Can you work these out from the model? Positions are in its coordinate system, mm. A direction names the side the tool comes from. Give positions to 0.01 mm unless a question says otherwise; leave off trailing zeros. Loops run counter-clockwise (first coordinate to the right, second up) from the corner with the lowest first, then second, coordinate; pieces in that order, holes last. Notation, with made-up numbers: (30.25, -28) -> (48.25, -28) arc R14 ccw to (48.25, -20) -> close; hole circle Ø5 at (-13.5, -8). An arc over 180 degrees is marked (long way). Use CSV: the item, a comma, the result in double quotes.
from build123d import *

# Parameters (mm, degrees)
SKETCH1_R           = 10.922
EXTRUDE1_DEPTH      = 94.869
EXTRUDE1_DEPTH_BACK = 94.869
SKETCH3_W           = 0.762
SKETCH3_H           = 0.762
RODHOLE_START       = -173.569
SKETCH8_R           = 3.175
RODHOLE_DEPTH       = 173.569
SKETCH9_R           = 9.525
STROKECHAMBER_DEPTH = 132
CHAMFER1_SIZE       = 0.5
SKETCH4_W           = 1.397
SKETCH4_H           = 12.7
SKETCH4_W_2         = 3.048
SKETCH4_H_2         = 3.048
FLATS_DEPTH         = 11.9220001
FLATS_DEPTH_BACK    = 11.9220001


with BuildPart() as part:
    # Sketch1 → Extrude1 (new body, two sides)
    with BuildSketch(Plane.XY) as extrude1_sk:
        Circle(SKETCH1_R)
    extrude(amount=EXTRUDE1_DEPTH)
    extrude(extrude1_sk.sketch, amount=-EXTRUDE1_DEPTH_BACK)

    # Sketch2 → Nose (revolve)
    with BuildSketch(Plane(origin=(0, 0, 0), x_dir=(0, 0, -1), z_dir=(1, 0, 0))):
        Polygon((-94.869, 7.9248), (-97.155, 7.9248), (-97.155, 7), (-99.955, 7), (-99.955, 7.9375), (-107.569, 7.9375), (-107.569, 0), (-94.869, 0), align=None)
    revolve(axis=Axis((0, 0, 0), (0, 0, 1)))

    # Sketch3 → CoverGrooves (revolve, cut)
    with BuildSketch(Plane(origin=(0, 0, 0), x_dir=(0, 0, -1), z_dir=(1, 0, 0))):
        with Locations((-75.438, 10.541)):
            Rectangle(SKETCH3_W, SKETCH3_H)
        Polygon((-74.295, 10.922), (-74.295, 10.16), (-73.533, 10.16), (-72.771, 10.922), align=None)
        Polygon((88.646, 10.922), (88.646, 10.16), (87.884, 10.922), align=None)
        Polygon((87.122, 10.922), (87.122, 10.16), (86.36, 10.922), align=None)
    revolve(axis=Axis((0, 0, 0), (0, 0, 1)), mode=Mode.SUBTRACT)

    # Sketch7 → FrontPort (revolve, cut)
    with BuildSketch(Plane(origin=(0, 0, 0), x_dir=(0, 0, -1), z_dir=(1, 0, 0))):
        Polygon((-83.439, 10.922), (-77.589, 10.922), (-78.289, 10.222), (-78.289, 0), (-83.439, 0), align=None)
    revolve(axis=Axis((0, 0, 83.439), (0, 1, 0)), mode=Mode.SUBTRACT)

    # Sketch8 → RodHole (cut)
    with BuildSketch(Plane.XY.offset(107.569).offset(RODHOLE_START)):
        Circle(SKETCH8_R)
    extrude(amount=RODHOLE_DEPTH, mode=Mode.SUBTRACT)

    # Sketch9 → StrokeChamber (cut)
    with BuildSketch(Plane.XY.offset(-66)):
        Circle(SKETCH9_R)
    extrude(amount=STROKECHAMBER_DEPTH, mode=Mode.SUBTRACT)

    # Chamfer1
    chamfer1_edges = [part.edges().sort_by_distance(p)[0] for p in [
        (-10.922, 0, -94.869),
        (-3.175, 0, 107.569),
        (0, -7.9375, 107.569),
        (-10.922, 0, 94.869),
    ]]
    chamfer(chamfer1_edges, length=CHAMFER1_SIZE)

    # Sketch4 → Flats (cut, two sides)
    with BuildSketch(Plane(origin=(0, 0, 0), x_dir=(1, 0, 0), z_dir=(0, 1, 0))) as flats_sk:
        with Locations((10.2235, -88.519)):
            Rectangle(SKETCH4_W, SKETCH4_H)
        with Locations((9.398, 93.345)):
            Rectangle(SKETCH4_W_2, SKETCH4_H_2)
        with Locations((-9.398, 93.345)):
            Rectangle(SKETCH4_W_2, SKETCH4_H_2)
        with Locations((-10.2235, -88.519)):
            Rectangle(SKETCH4_W, SKETCH4_H)
    extrude(amount=FLATS_DEPTH, mode=Mode.SUBTRACT)
    extrude(flats_sk.sketch, amount=-FLATS_DEPTH_BACK, mode=Mode.SUBTRACT)

    # Sketch10 → RearStdPort (revolve, cut)
    with BuildSketch(Plane(origin=(0, 0, 0), x_dir=(0, 0, -1), z_dir=(1, 0, 0))):
        Polygon((94.869, 0), (94.869, 5.85), (94.169, 5.15), (0, 5.15), (0, 0), align=None)
    revolve(axis=Axis((0, 0, 0), (0, 0, 1)), mode=Mode.SUBTRACT)


solid = part.part
(1) If we section it at C-C, the plane z = -33: Write out the boundary of the cut face in (x, y) (3 decimals), then the cut area to 3 significant figures.
Answer sheet:
outline,"circle Ø21.844 at (0, 0); hole circle Ø19.05 at (0, 0)"
area,"89.7 mm2"
(2) If we section it at D-D, the plane z = -73: Write out the boundary of the cut face in (x, y), then the cut area to 3 significant figures.
Answer sheet:
outline,"circle Ø21.84 at (0, 0); hole circle Ø10.3 at (0, 0)"
area,"291 mm2"
(3) If we section it at A-A, the plane z = 92: Write out the boundary of the cut face in (x, y) (3 decimals), then the cut area to 3 significant figures.
Answer sheet:
outline,"(-9.525, -5.345) arc R10.922 ccw to (9.525, -5.345) -> (9.525, 5.345) arc R10.922 ccw to (-9.525, 5.345) -> close; hole circle Ø6.35 at (0, 0)"
area,"323 mm2"
(4) Which directions (+Z, -Z, +X, -X, +Y, -Y) give clear straight access to the entire face, cutting with the end or side of a thin tool? Please do faces 1 (the face through (4, 0, 66)), 2 (the face through (9.525, 0, 89)), 3 (the face through (-0.226, 5.039, 88.584)).
Answer sheet:
face 1,"none"
face 2,"+Z, +X, +Y, -Y"
face 3,"+Y"
(5) If we section it at B-B, the plane x = 0: Give the number of separate pieces and of enclosed holes in the cut face, then the cut area to 3 significant figures.
Answer sheet:
separate pieces,"3"
enclosed holes,"0"
area,"1,180 mm2"
(6) We'd pull the mould along Z, two halves only. Please class faces 4 (the face through (10.09, -4.18, 74.68)), 5 (the face through (-7.559, -5.796, -0.924)), 6 (the face through (0.17, 10.56, 94.73)): released by +Z, released by -Z, zero draft, split by the parting line, or undercut.
Answer sheet:
face 4,"zero draft"
face 5,"undercut"
face 6,"released by +Z"
(7) Will these pins go through, and if not, where does the flat tip stop? pin 1 Ø6 at (y, z) = (7.5, 51.5) entering from -X; pin 2 Ø1.6 at (x, z) = (4, 85.5) entering from +Y; pin 3 Ø1.6 at (x, z) = (-4, 82.5) entering from +Y.
Answer sheet:
pin 1,"stops at x = -9.95"
pin 2,"stops at y = 10.03"
pin 3,"stops at y = 0"
(8) If I drill on L1, parallel to Z at x = 1, y = 9; L2, parallel to Z at x = 9, y = -5.5 (3 decimals); L3, parallel to Z at x = 0, y = 5, over which ranges is the centre line in solid material (lowest first)? Write a range as from..to.
Answer sheet:
L1,"z = -94.87..-66, 66..78.39, 88.49..94.87"
L2,"z = -91.821..-88.646, -88.258..-87.122, -86.734..73.145, 74.295..75.057, 75.819..94.743"
L3,"z = 66..78.29, 88.59..107.57"
